Geometry check sheet. Reference: the model listing, model coordinates, mm. A direction names the side the tool comes from. Give positions to 0.01 mm unless a question says otherwise; leave off trailing zeros. Write each loop counter-clockwise with the first axis right and the second up, starting at its lowest first coordinate (ties: lowest second). Pieces come first, ordered by that corner, then holes. Notation, with made-up numbers: (73.25, -4) - (110.25, -4) arc R12 cw to (110.25, 14) - close; hole circle Ø7 at (-1.75, -27.5). An arc over 180 degrees is marked (long way). Use a Markdown table: item, result.
```python
from build123d import *

# Parameters (mm, degrees)
EXTRUDE_THIN1_DEPTH = 508
CAVITY2_START       = 209.868015847
CAVITY2_DEPTH       = 76.2


# Read off the part's stored shape, not the designer's step: Cavity2
with BuildPart() as part:
    # Sketch1 → Extrude-Thin1 (new body)
    with BuildSketch(Plane(origin=(0, 0, 0), x_dir=(0, 0, -1), z_dir=(1, 0, 0))):
        with BuildLine():
            ThreePointArc((0, 660.4), (-660.4, 0), (0, -660.4))
            Line((0, -660.4), (0, -711.2))
            ThreePointArc((0, -711.2), (-711.2, 0), (0, 711.2))
            Line((0, 711.2), (0, 660.4))
        make_face()
    extrude(amount=EXTRUDE_THIN1_DEPTH)

    # Cavity2 outline → Cavity2 (cut)
    with BuildSketch(Plane.YZ.offset(CAVITY2_START)):
        with BuildLine():
            ThreePointArc((706.028233309, 0), (2.092834501, 668.954640909), (-701.842564308, 0))
            Line((-701.842564308, 0), (-660.4, 0))
            ThreePointArc((-660.4, 0), (0, 660.4), (660.4, 0))
            Line((660.4, 0), (706.028233309, 0))
        make_face()
    extrude(amount=CAVITY2_DEPTH, mode=Mode.SUBTRACT)


solid = part.part
```
1) Mould release check, pull along X, two halves, no side actions. Record for faces 3 (the cylindrical face through (247.435, 17.089, 668.795)), 4 (the cylindrical face through (103.46, 14.52, 660.24)), 5 (the flat face through (508, 3, 670)): pulls with the +X half, pulls with the -X half, needs draft (parallel to the pull), parting line crosses it, or undercut.
Working result:
| item | result |
|---|---|
| face 3 | undercut |
| face 4 | needs draft |
| face 5 | pulls with the +X half |
2) Section check A-A on z = 193. Record the boundary of the cut face in (x, y).
Working result:
| item | result |
|---|---|
| outline | (0, -684.51) - (508, -684.51) - (508, -631.57) - (286.07, -631.57) - (286.07, -664.56) - (209.87, -664.56) - (209.87, -631.57) - (0, -631.57) - close; (0, 631.57) - (209.87, 631.57) - (209.87, 668.74) - (286.07, 668.74) - (286.07, 631.57) - (508, 631.57) - (508, 684.51) - (0, 684.51) - close |
3) Set-up check for faces 1 (the flat face through (286.068, 103, 658)), 2 (the flat face through (250, -702, 0)): record each of +Z, -Z, +X, -X, +Y, -Y from which the full face is reachable in a straight line by a thin tool's end or side.
Working result:
| item | result |
|---|---|
| face 1 | -Z |
| face 2 | -Z, +X, -X, +Y, -Y |
4) Section check B-B on y = 60. Record the boundary of the cut face in (x, z), then the cut area to 3 significant figures.
Working result:
| item | result |
|---|---|
| outline | (0, 657.67) - (209.87, 657.67) - (209.87, 666.57) - (286.07, 666.57) - (286.07, 657.67) - (508, 657.67) - (508, 708.66) - (0, 708.66) - close |
| area | 25,200 mm² |
5) Section check C-C on z = 517. Record the boundary of the cut face in (x, y).
Working result:
| item | result |
|---|---|
| outline | (0, -488.38) - (508, -488.38) - (508, -410.9) - (286.07, -410.9) - (286.07, -435.08) - (209.87, -435.08) - (209.87, -410.9) - (0, -410.9) - close; (0, 410.9) - (209.87, 410.9) - (209.87, 439.27) - (286.07, 439.27) - (286.07, 410.9) - (508, 410.9) - (508, 488.38) - (0, 488.38) - close |
6) Material ranges on L1, parallel to Z at x = 288.5, y = 7; L2, parallel to Y at x = 418.5, z = 337.5; L3, parallel to Y at x = 62, z = 177.5, recorded low to high. Write a range as from..to.
Working result:
| item | result |
|---|---|
| L1 | z = 660.36..711.17 |
| L2 | y = -626.02..-567.65, 567.65..626.02 |
| L3 | y = -688.69..-636.1, 636.1..688.69 |
7) Depth check by flat-ended pin: P1, Ø6, axis at x = 314, z = 183, coming from the -Y side; P2, Ø5, axis at x = 291, y = -463.5, coming from the +Z side; P3, Ø5, axis at x = 203.5, z = 140.5, coming from the -Y side. Enter the tip coordinate at first touch or a pass-through.
Working result:
| item | result |
|---|---|
| P1 | stops at y = -688.04 |
| P2 | stops at z = 541.56 |
| P3 | stops at y = -697.68 |
8) Section check D-D on x = 477. Record the boundary of the cut face in (y, z).
Working result:
| item | result |
|---|---|
| outline | (-711.2, 0) - (-660.4, 0) arc R660.4 cw to (660.4, 0) - (711.2, 0) arc R711.2 ccw to start |
